For this review, take the finished solid that the model builds, in its own axes (mm). A direction names the side the tool comes from. Give positions to 0.01 mm unless a question says otherwise; leave off trailing zeros. Write each loop counter-clockwise with the first axis right and the second up, starting at its lowest first coordinate (ties: lowest second). Pieces come first, ordered by that corner, then holes.
1) Machinability: for faces 1 (the face through (5.225, 0.891, 2.007)), 2 (the face through (0.175, 26.314, 1.268)), 3 (the face through (-2, -1, 0)), 4 (the face through (17.21, 2.1, 1.23)), 5 (the face through (-8.13, -15.58, 1.23)), which of the approach directions +Z, -Z, +X, -X, +Y, -Y give a long, thin tool a straight path to every point of the face, cutting with its end or side? Answer none if there is none.
2) We need section A-A on x = -15. Give the boundary of the cut face in (y, z).
3) For P1, Ø1.1, axis at x = 1.5, z = 2, coming from the +Y side; P2, Ø0.5, axis at x = -1, z = 2, coming from the -Y side; P3, Ø1, axis at y = 14, z = 2, coming from the +X side, all flat-tipped, find the tip position at first contact; note any pin that passes through.
4) We need section B-B on z = 0.8. Give the boundary of the cut face in (x, y).
5) Draft analysis for pull direction X (two halves, no side actions). For faces 6 (the face through (-17.33, 2.92, 1.23)), 7 (the face through (-1.4, 0.6, 1.5)), 8 (the face through (0, 3, 2.5)), state which applies: pulls with the +X half, pulls with the -X half, needs draft (parallel to the pull), parting line crosses it, or undercut.
6) We need section C-C on y = 16. Give the boundary of the cut face in (x, z), and give its area (3 significant figures).
7) Wall thickness on line 1 along X through (y, z) = (-11, 1.1); line 2 along X through (y, z) = (-10.5, 0.6); line 3 along Y through (x, z) = (17, 0.5): over which ranges is each line inside the solid? List them lowest first.
8) We need section D-D on x = -9. Give the boundary of the cut face in (y, z).
from build123d import *

# Parameters (mm, degrees)
EXTRUDE_1_DEPTH     = 2.5
CUT_EXTRUDE_1_DEPTH = 1
SKETCH_4_R          = 1.5
CUT_EXTRUDE_3_DEPTH = 2.5


with BuildPart() as part:
    # 草图1 → 凸台-拉伸1 (new body)
    with BuildSketch(Plane.XY):
        with BuildLine():
            Line((-24.844384519, 8.60192761), (-9.608590106, -2.919770039))
            Line((-9.608590106, -2.919770039), (-15.858256337, -20.970271974))
            Line((-15.858256337, -20.970271974), (-0.192351313, -10.040570794))
            Line((-0.192351313, -10.040570794), (15.0434431, -21.562268443))
            Line((15.0434431, -21.562268443), (9.487934055, -3.286883328))
            Line((9.487934055, -3.286883328), (25.155615481, 7.644057202))
            Line((25.155615481, 7.644057202), (6.053810642, 8.009998274))
            Line((6.053810642, 8.009998274), (0.799130777, 25.295776665))
            ThreePointArc((0.799130777, 25.295776665), (0.520604646, 30.277806022), (0.162308714, 25.300877517))
            Line((0.162308714, 25.300877517), (-5.746083956, 8.236053671))
            Line((-5.746083956, 8.236053671), (-24.844384519, 8.60192761))
        make_face()
    extrude(amount=EXTRUDE_1_DEPTH)

    # 草图2 → 切除-拉伸1 (cut)
    with BuildSketch(Plane.XY.offset(2.5)):
        with BuildLine():
            Line((-3.743094252, 1.70920022), (-4.057196816, 1.468815604))
            add(Edge.make_bspline(
                [(-4.057196816, 1.468815604), (-4.079603546, 1.49551957), (-4.124114914, 1.548567474), (-4.195725431, 1.623058382), (-4.27035588, 1.692847252), (-4.347977733, 1.758266543), (-4.429988155, 1.817028561), (-4.514400496, 1.872195536), (-4.602626834, 1.921644379), (-4.724628816, 1.981602077), (-4.884226357, 2.044169112), (-5.085134745, 2.096629947), (-5.294861714, 2.130025577), (-5.437944685, 2.133642538), (-5.510722457, 2.135482271)],
                knots=[0, 0, 0, 0, 0.757959112, 1.505699292, 2.245454638, 2.979532153, 3.711538275, 4.438200793, 5.171680507, 5.909471876, 7.393775596, 8.890124382, 10.418191784, 12, 12, 12, 12], degree=3))
            add(Edge.make_bspline(
                [(-5.510722457, 2.135482271), (-5.550817657, 2.1350206), (-5.630635934, 2.134101541), (-5.749091332, 2.121976827), (-5.865334819, 2.104935444), (-5.979290781, 2.07964936), (-6.090814162, 2.047680653), (-6.20063405, 2.00948018), (-6.30716045, 1.962217506), (-6.411867008, 1.909979494), (-6.512186106, 1.8509767), (-6.60710616, 1.786618584), (-6.696280981, 1.717625331), (-6.779781109, 1.643738352), (-6.857691907, 1.565290397), (-6.929448834, 1.481445435), (-6.994803588, 1.392471523), (-7.055051617, 1.299541914), (-7.109009027, 1.202927295), (-7.154186032, 1.102270072), (-7.194191886, 0.999293954), (-7.225848163, 0.892835485), (-7.250904753, 0.783643752), (-7.268193512, 0.671425709), (-7.280180336, 0.556415789), (-7.281094824, 0.478462289), (-7.281555791, 0.439168169)],
                knots=[0, 0, 0, 0, 1.054917814, 2.100044995, 3.131103042, 4.146048494, 5.169673617, 6.183595914, 7.203665975, 8.234915748, 9.262203917, 10.264457458, 11.251630812, 12.227803204, 13.197192746, 14.159520551, 15.12972552, 16.100847026, 17.073214652, 18.039054194, 19.002613845, 19.979014051, 20.95965708, 21.949030935, 22.966165397, 24, 24, 24, 24], degree=3))
            add(Edge.make_bspline(
                [(-7.281555791, 0.439168169), (-7.280113712, 0.38004666), (-7.277282381, 0.26396942), (-7.252084285, 0.093945865), (-7.213792752, -0.068934905), (-7.156403521, -0.223654725), (-7.085638892, -0.372121419), (-6.996221051, -0.511822966), (-6.892659294, -0.644870468), (-6.773488528, -0.768119552), (-6.642739024, -0.880706666), (-6.502455697, -0.979850188), (-6.352987939, -1.062495768), (-6.195986076, -1.131268278), (-6.030241946, -1.18413311), (-5.856053601, -1.221349251), (-5.673799892, -1.245626029), (-5.549263435, -1.247950244), (-5.485882714, -1.249133114)],
                knots=[0, 0, 0, 0, 1.029171465, 2.020641659, 2.987623507, 3.938342917, 4.889210282, 5.84687017, 6.821220943, 7.821438502, 8.827599549, 9.822697543, 10.807740252, 11.797342354, 12.80366471, 13.83203677, 14.896651826, 16, 16, 16, 16], degree=3))
            add(Edge.make_bspline(
                [(-5.485882714, -1.249133114), (-5.416051069, -1.24720308), (-5.278605688, -1.243404311), (-5.077042229, -1.211222312), (-4.884087068, -1.159041834), (-4.699729826, -1.086015637), (-4.524490231, -0.99108388), (-4.358094048, -0.876000591), (-4.200400824, -0.739671068), (-4.105576502, -0.635576065), (-4.057196816, -0.582466447)],
                knots=[0, 0, 0, 0, 1.028121516, 2.023589091, 2.998037872, 3.967518031, 4.937445131, 5.927275754, 6.942489185, 8, 8, 8, 8], degree=3))
            Line((-4.057196816, -0.582466447), (-3.743094252, -0.820447216))
            add(Edge.make_bspline(
                [(-3.743094252, -0.820447216), (-3.768372092, -0.85306259), (-3.818806692, -0.918137111), (-3.900472998, -1.009876208), (-3.986504195, -1.096166534), (-4.077539292, -1.176312387), (-4.172531054, -1.251917491), (-4.273185125, -1.320833869), (-4.378178305, -1.384023451), (-4.487154852, -1.441882794), (-4.599998981, -1.49321679), (-4.716575478, -1.537163953), (-4.83638185, -1.57502097), (-4.959423574, -1.606166041), (-5.085955868, -1.630475851), (-5.215522124, -1.646726908), (-5.348401981, -1.657860524), (-5.438049319, -1.658875285), (-5.483478868, -1.659389524)],
                knots=[0, 0, 0, 0, 0.986787822, 1.968848986, 2.935600012, 3.899624008, 4.868462664, 5.837806735, 6.815139263, 7.798259679, 8.787526145, 9.778297419, 10.776456485, 11.791383307, 12.812564526, 13.85620153, 14.913611965, 16, 16, 16, 16], degree=3))
            add(Edge.make_bspline(
                [(-5.483478868, -1.659389524), (-5.526500201, -1.659090104), (-5.611569562, -1.658498038), (-5.737168135, -1.648906989), (-5.859441941, -1.635821576), (-5.978041514, -1.616118569), (-6.093614057, -1.592867894), (-6.205111868, -1.561700744), (-6.313632108, -1.526787411), (-6.418738783, -1.48575314), (-6.520521297, -1.439448931), (-6.618651367, -1.387115721), (-6.713083861, -1.32919359), (-6.8047472, -1.266959293), (-6.892287295, -1.198413805), (-6.976462753, -1.12450908), (-7.057745583, -1.04549421), (-7.108034366, -0.988517235), (-7.133318611, -0.959870293)],
                knots=[0, 0, 0, 0, 1.114604814, 2.203992996, 3.262667896, 4.300477797, 5.318619304, 6.316056647, 7.298880507, 8.271930387, 9.238335007, 10.195173496, 11.151986948, 12.108099108, 13.064862484, 14.031167946, 15.010108607, 16, 16, 16, 16], degree=3))
            add(Edge.make_bspline(
                [(-7.133318611, -0.959870293), (-7.17381649, -0.910108934), (-7.25432332, -0.81118698), (-7.357324101, -0.650860144), (-7.445492736, -0.483467905), (-7.516779503, -0.308130844), (-7.57250834, -0.125242401), (-7.61111542, 0.065289615), (-7.636202968, 0.263287264), (-7.63907187, 0.397957879), (-7.64053015, 0.466411758)],
                knots=[0, 0, 0, 0, 0.994628077, 1.977248131, 2.950237994, 3.925870899, 4.908910175, 5.911660606, 6.938484602, 8, 8, 8, 8], degree=3))
            add(Edge.make_bspline(
                [(-7.64053015, 0.466411758), (-7.638752786, 0.538360848), (-7.635255933, 0.67991619), (-7.605546452, 0.887657851), (-7.557753542, 1.086688021), (-7.489871384, 1.276635158), (-7.403808125, 1.458498335), (-7.297491995, 1.630888284), (-7.172158118, 1.794907483), (-7.02878947, 1.948067199), (-6.871569658, 2.088112174), (-6.703205299, 2.211319264), (-6.524025931, 2.313853568), (-6.336005529, 2.399563468), (-6.137736179, 2.465442854), (-5.9296409, 2.511560782), (-5.712110712, 2.540266057), (-5.563696511, 2.543894866), (-5.48828656, 2.545738681)],
                knots=[0, 0, 0, 0, 1.032925535, 2.032216505, 3.007276963, 3.968222605, 4.92396291, 5.891752235, 6.871517503, 7.883894988, 8.900124299, 9.891468569, 10.874487609, 11.85992873, 12.854644235, 13.869047385, 14.917252991, 16, 16, 16, 16], degree=3))
            add(Edge.make_bspline(
                [(-5.48828656, 2.545738681), (-5.442327163, 2.545187666), (-5.351355167, 2.544096987), (-5.216780707, 2.533461396), (-5.085760904, 2.515731561), (-4.958205496, 2.49159891), (-4.833493935, 2.461647685), (-4.712579374, 2.422630201), (-4.594752303, 2.378017023), (-4.480755837, 2.326635919), (-4.371136922, 2.268959643), (-4.265929701, 2.205627502), (-4.165969863, 2.13671801), (-4.070554036, 2.062817238), (-3.981278366, 1.982361741), (-3.895608105, 1.897564489), (-3.816452587, 1.805982975), (-3.767591793, 1.741520194), (-3.743094252, 1.70920022)],
                knots=[0, 0, 0, 0, 1.096760587, 2.17092713, 3.219439832, 4.250915756, 5.268269357, 6.278326846, 7.281116186, 8.274029601, 9.260640565, 10.235837813, 11.203064059, 12.156899882, 13.114053108, 14.069676657, 15.032185724, 16, 16, 16, 16], degree=3))
        make_face()
        Polygon((-2.922581432, 2.443174579), (-2.563607073, 2.443174579), (-2.563607073, 0.802148938), (-0.512325021, 0.802148938), (-0.512325021, 2.443174579), (-0.153350663, 2.443174579), (-0.153350663, -1.556825421), (-0.512325021, -1.556825421), (-0.512325021, 0.391892527), (-2.563607073, 0.391892527), (-2.563607073, -1.556825421), (-2.922581432, -1.556825421), align=None)
        Polygon((0.872290363, 2.443174579), (3.12870062, 2.443174579), (3.12870062, 2.032918169), (1.231264722, 2.032918169), (1.231264722, 0.802148938), (3.12870062, 0.802148938), (3.12870062, 0.391892527), (1.231264722, 0.391892527), (1.231264722, -1.146569011), (3.12870062, -1.146569011), (3.12870062, -1.556825421), (0.872290363, -1.556825421), align=None)
        Polygon((3.846649337, -1.556825421), (3.846649337, 2.443174579), (3.92196985, 2.443174579), (6.564598055, -0.705062601), (6.564598055, 2.443174579), (6.923572414, 2.443174579), (6.923572414, -1.556825421), (6.841841645, -1.556825421), (4.205623696, 1.58420022), (4.205623696, -1.556825421), align=None)
    extrude(amount=-CUT_EXTRUDE_1_DEPTH, mode=Mode.SUBTRACT)

    # 草图4 → 切除-拉伸3 (cut)
    with BuildSketch(Plane.XY.offset(2.5)):
        with Locations((0.500580653, 27.777886216)):
            Circle(SKETCH_4_R)
    extrude(amount=-CUT_EXTRUDE_3_DEPTH, mode=Mode.SUBTRACT)


solid = part.part
Results list:
1. face 1: +Z
1. face 2: +Z, -Z
1. face 3: -Z, +X, -X, +Y, -Y
1. face 4: +Z, -Z, +X
1. face 5: +Z, -Z, -Y
2. outline: (-20.37, 0) - (-18.49, 0) - (-18.49, 2.5) - (-20.37, 2.5) - close; (1.16, 0) - (8.41, 0) - (8.41, 2.5) - (1.16, 2.5) - close
3. P1: stops at y = 30.24
3. P2: stops at y = -10.78
3. P3: stops at x = 4.38
4. outline: (-24.84, 8.6) - (-9.61, -2.92) - (-15.86, -20.97) - (-0.19, -10.04) - (15.04, -21.56) - (9.49, -3.29) - (25.16, 7.64) - (6.05, 8.01) - (0.8, 25.3) arc R2.5 ccw (long way) to (0.16, 25.3) - (-5.75, 8.24) - close; hole circle Ø3 at (0.5, 27.78)
5. face 6: pulls with the -X half
5. face 7: undercut
5. face 8: needs draft
6. outline: (-3.06, 0) - (3.62, 0) - (3.62, 2.5) - (-3.06, 2.5) - close
6. area: 16.7 mm2
7. line 1: x = -12.41 to -1.57, 1.08 to 11.83
7. line 2: x = -12.23 to -0.85, 0.42 to 11.68
7. line 3: y = 1.95 to 7.8
8. outline: (-16.19, 0) - (8.3, 0) - (8.3, 2.5) - (-16.19, 2.5) - close
